```python
from build123d import *

# Parameters (mm, degrees)
CHAMFER1_SIZE = 0.5


with BuildPart() as part:
    # Sketch1 → Revolve1 (revolve)
    with BuildSketch(Plane.XY, mode=Mode.PRIVATE) as revolve1_sk:
        Polygon((0, 22.5), (110, 22.5), (110, 17), (64, 17), (64, 12), (4, 12), (4, 9), (0, 9), align=None)
    revolve(revolve1_sk.sketch.rotate(Axis((0, 0, 0), (1, 0, 0)), 90), axis=Axis((0, 0, 0), (1, 0, 0)))

    # Chamfer1
    chamfer1_edges = [part.edges().sort_by_distance(p)[0] for p in [
        (0, 0, -22.5),
        (0, 0, -9),
        (64, 0, -17),
        (110, 0, -17),
        (110, 0, -22.5),
    ]]
    chamfer(chamfer1_edges, length=CHAMFER1_SIZE)


solid = part.part
```
Part model, mm, in its own coordinate system. A direction names the side the tool comes from. Give positions to 0.01 mm unless a question says otherwise; leave off trailing zeros. Write each loop counter-clockwise with the first axis right and the second up, starting at its lowest first coordinate (ties: lowest second). Pieces come first, ordered by that corner, then holes. Notation, with made-up numbers: (55, 70.25) -> (83, 70.25) arc R16 cw to (83, 80.25) -> close; hole circle Ø8 at (2.25, -2.75). An arc over 180 degrees is marked (long way). Put each result on its own line as item: value. Start each with the question number.
Item 1: Cut at C-C (x = 49). List the corners of the cut face in (y, z).
Item 2: Which spindle directions (+Z, -Z, +X, -X, +Y, -Y) get a long thin tool onto all of the face, cutting with end or side? Do faces 4 (the face through (110, 10, -15)), 5 (the face through (86.685, -16.855, -2.213)). Say none if no direction does.
Item 3: Pull direction Z, two halves, no side cores. Call faces 1 (the face through (2.226, -6.083, -6.633)), 2 (the face through (0, 5, -9)), 3 (the face through (55.763, 19.961, 10.382)): pulls with the +Z half, pulls with the -Z half, needs draft (parallel to the pull), parting line crosses it, or undercut.
Item 4: Cut at A-A (y = 0). List the corners of the cut face in (x, z), then the cut area to 3 significant figures.
Item 5: Pin check, flat tips, straight feed: pin 1 Ø1.5 at (x, z) = (76, -12.5) entering from -Y; pin 2 Ø7 at (y, z) = (2.5, 5.5) entering from +X; pin 3 Ø12 at (x, y) = (37.5, -8.5) entering from -Z; pin 4 Ø8 at (y, z) = (1.5, -14) entering from -X. Stop position of each tip, or through.
Item 6: Cut at D-D (x = 95). List the corners of the cut face in (y, z), then the cut area to 3 significant figures.
Item 7: Wall check: L1, parallel to Y at x = 30, z = 0; L2, parallel to Y at x = 3.2, z = 0; L3, parallel to X at y = 0, z = -15.5. Give the ranges that are in metal, low to high. Write a range as [from, to].
Answer list:
1. outline: circle Ø45 at (0, 0); hole circle Ø24 at (0, 0)
2. face 4: +Z, -Z, +X, +Y, -Y
2. face 5: +X
3. face 1: undercut
3. face 2: needs draft
3. face 3: parting line crosses it
4. outline: (0, -22) -> (0.5, -22.5) -> (109.5, -22.5) -> (110, -22) -> (110, -17.5) -> (109.5, -17) -> (64.5, -17) -> (64, -16.5) -> (64, -12) -> (4, -12) -> (4, -9) -> (0.5, -9) -> (0, -9.5) -> close; (0, 9.5) -> (0.5, 9) -> (4, 9) -> (4, 12) -> (64, 12) -> (64, 16.5) -> (64.5, 17) -> (109.5, 17) -> (110, 17.5) -> (110, 22) -> (109.5, 22.5) -> (0.5, 22.5) -> (0, 22) -> close
4. area: 1,870 mm2
5. pin 1: stops at y = -19.19
5. pin 2: stops at x = 4
5. pin 3: stops at z = -22.36
5. pin 4: stops at x = 0
6. outline: circle Ø45 at (0, 0); hole circle Ø34 at (0, 0)
6. area: 683 mm2
7. L1: y = [-22.5, -12], [12, 22.5]
7. L2: y = [-22.5, -9], [9, 22.5]
7. L3: x = [0, 64]
